```python
from build123d import *

# Parameters (mm, degrees)
SKETCH_1_R               = 2.95
EXTRUDE_1_DEPTH          = 1.2
SKETCH_2_R               = 2
EXTRUDE_2_DEPTH          = 1.9
CUT_EXTRUDE_1_DEPTH      = 0.5
PATTERN_CIRCULAR_1_COUNT = 20
SKETCH_4_W               = 0.35
SKETCH_4_H               = 0.5
SKETCH_6_W               = 8.9
SKETCH_6_H               = 2
CHAMFER_2_SIZE           = 0.5
CUT_EXTRUDE_START        = -0.5
SKETCH_7_R               = 2.95
SKETCH_7_R_2             = 2.75
CUT_EXTRUDE_2_DEPTH      = 0.5
CHAMFER_3_SIZE           = 0.25


with BuildPart() as part:
    # Эскиз1 → Вытянуть1 (new body)
    with BuildSketch(Plane.XY):
        Circle(SKETCH_1_R)
    extrude(amount=EXTRUDE_1_DEPTH)

    # Эскиз2 → Вытянуть2 (add)
    with BuildSketch(Plane.XY.offset(1.2)):
        with Locations(Location((0, 0, 0), (0, 0, 180))):
            Circle(SKETCH_2_R)
    extrude(amount=EXTRUDE_2_DEPTH)

    # Эскиз3 → Вырез-Вытянуть1 (cut)
    with BuildSketch(Plane.XY.offset(1.2)):
        Polygon((-0.393502884, 2.95), (0.393502884, 2.95), (0, 2), align=None)
    cut_extrude_1 = extrude(amount=-CUT_EXTRUDE_1_DEPTH, mode=Mode.SUBTRACT)

    # Круговой массив1: Вырез-Вытянуть1 ×20 about axis
    pattern_circular_1_axis = Axis((0, 0, 0), (0, 0, 1))
    for i in range(1, PATTERN_CIRCULAR_1_COUNT):
        add(cut_extrude_1.rotate(pattern_circular_1_axis, i * 360 / PATTERN_CIRCULAR_1_COUNT), mode=Mode.SUBTRACT)

    # Эскиз4 → Вырез-Повернуть1 (revolve, cut)
    with BuildSketch(Plane(origin=(0, 0, 0), x_dir=(1, 0, 0), z_dir=(0, 1, 0)), mode=Mode.PRIVATE) as cut_revolve_1_sk:
        with Locations((1.825, -2.25)):
            Rectangle(SKETCH_4_W, SKETCH_4_H)
    revolve(cut_revolve_1_sk.sketch.rotate(Axis((0, 0, 14.805168786), (0, 0, -1)), 172.537215717), axis=Axis((0, 0, 14.805168786), (0, 0, -1)), mode=Mode.SUBTRACT)

    # Эскиз6 → Повернуть1 (revolve)
    with BuildSketch(Plane(origin=(0, 0, 0), x_dir=(0, 0, -1), z_dir=(1, 0, 0)), mode=Mode.PRIVATE) as revolve_1_sk:
        with Locations((-7.55, -1)):
            Rectangle(SKETCH_6_W, SKETCH_6_H)
    revolve(revolve_1_sk.sketch.rotate(Axis((0, 0, 3.1), (0, 0, 1)), 277.462784283), axis=Axis((0, 0, 3.1), (0, 0, 1)))

    # Фаска2
    chamfer_2_edges = [part.edges().sort_by_distance(p)[0] for p in [
        (1.983058868, 0.25976437, 12),
    ]]
    chamfer(chamfer_2_edges, length=CHAMFER_2_SIZE)

    # Эскиз7 → Вырез-Вытянуть2 (cut)
    with BuildSketch(Plane.XY.offset(1.2).offset(CUT_EXTRUDE_START)):
        with Locations(Location((0, 0, 0), (0, 0, 180))):
            Circle(SKETCH_7_R)
        Circle(SKETCH_7_R_2, mode=Mode.SUBTRACT)
    extrude(amount=CUT_EXTRUDE_2_DEPTH, mode=Mode.SUBTRACT)

    # Фаска3
    chamfer_3_edges = [part.edges().sort_by_distance(p)[0] for p in [
        (2, 0, 2.5),
    ]]
    chamfer(chamfer_3_edges, length=CHAMFER_3_SIZE)


solid = part.part
```
The model under review builds one solid part; all positions refer to its coordinate system, in mm. A direction names the side the tool comes from. Coordinates: 2 decimals unless noted, no trailing zeros. Write each loop counter-clockwise with the first axis right and the second up, starting at its lowest first coordinate (ties: lowest second). Pieces come first, ordered by that corner, then holes.
1) We need section A-A on x = 2.15. State the section outline as (y, z) points.
2) Clearance check with flat-ended pins moving along their axes: pin 1 Ø2 at (y, z) = (2, 5) entering from -X; pin 2 Ø3 at (x, z) = (-0.5, 2.5) entering from +Y; pin 3 Ø0.7 at (x, y) = (0.5, 2.5) entering from +Z. State where each tip first meets the part, or that it passes through.
3) We need section B-B on z = 10.25. State the section outline as (x, y) points, then the cut area to 3 significant figures.
4) Machinability: for faces 1 (the face through (1.7, 1.6, 1.2)), 2 (the face through (1.6, -1.6, 1.2)), 3 (the face through (-1.6, -1.7, 1.2)), 4 (the face through (-1.904, -0.613, 7.064)), 5 (the face through (0, 0, 12)), which of the approach directions +Z, -Z, +X, -X, +Y, -Y give a long, thin tool a straight path to every point of the face, cutting with its end or side? Answer none if there is none.
5) To check wall thickness, follow probe 1 along Z at (x, y) = (1.3, 2.5); probe 2 along X at (y, z) = (0.75, 1.75); probe 3 along Y at (x, z) = (0.4, 5.5). State the ranges of each line that lie inside material, in increasing order.
6) The part is to be moulded in two halves that separate along Z. For faces 6 (the face through (-1.6, 1.6, 1.2)), 7 (the face through (-2.947, 0.13, 0.345)), 8 (the face through (0.56, -1.55, 2.25)), 9 (the face through (0, 0, 0)), say which applies: pulls with the +Z half, pulls with the -Z half, needs draft (parallel to the pull), parting line crosses it, or undercut.
Answer list:
1. outline: (-2.02, 0) - (2.02, 0) - (2.02, 0.7) - (1.3, 0.7) - (1.3, 1.2) - (0.83, 1.2) - (0.83, 0.7) - (0.6, 0.7) - (0.6, 1.2) - (0.06, 1.2) - (0.06, 0.7) - (-0.06, 0.7) - (-0.06, 1.2) - (-0.6, 1.2) - (-0.6, 0.7) - (-0.83, 0.7) - (-0.83, 1.2) - (-1.3, 1.2) - (-1.3, 0.7) - (-2.02, 0.7) - close
2. pin 1: stops at x = -1.73
2. pin 2: stops at y = 2.73
2. pin 3: stops at z = 1.2
3. outline: circle Ø4 at (0, 0)
3. area: 12.6 mm2
4. face 1: +Z, +X, +Y
4. face 2: +Z, +X, -Y
4. face 3: +Z, -X, -Y
4. face 4: +Z
4. face 5: +Z, +X, -X, +Y, -Y
5. probe 1: z = 0 to 0.7
5. probe 2: x = -1.85 to 1.85
5. probe 3: y = -1.96 to 1.96
6. face 6: pulls with the +Z half
6. face 7: needs draft
6. face 8: undercut
6. face 9: pulls with the -Z half
